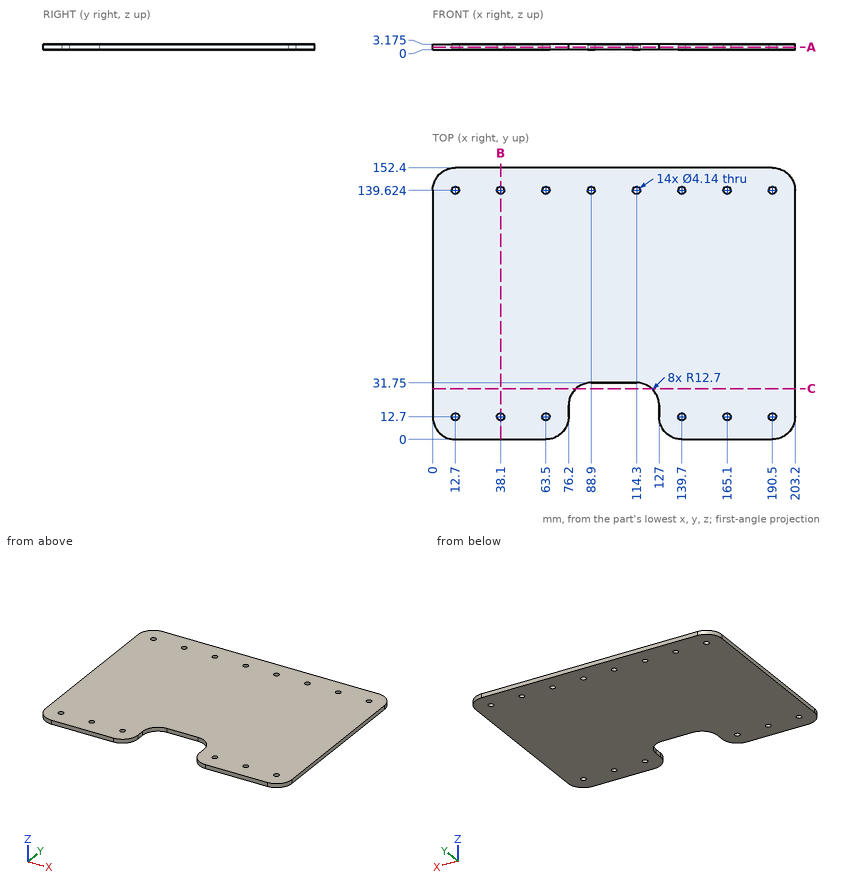
Source: three-view drawing plus pictorial views. Frame: mm from the lowest corner of the part. Round coordinates to 2 decimals unless told otherwise and drop trailing zeros. Write each loop counter-clockwise with the first axis right and the second up, starting at its lowest first coordinate (ties: lowest second). Pieces come first, ordered by that corner, then holes. Notation, with made-up numbers: M -20,34.25 L -2,34.25 A19 ccw -2,64.25 Z; hole C -29,46.25 d9. An arc over 180 degrees is marked long. One line per item, written item: value. Start each with the question number.
Item 1: Section query A-A (z = 1.35). State how many separate pieces and enclosed holes the cut face has, plus the area to 3 significant figures.
Item 2: Section query C-C (y = 28.5). Return the cut outline in (x, z) (1 decimal).
Item 3: Section query B-B (x = 38.1). Return the cut outline in (y, z) (1 decimal).
Item 4: Ray query, L1, parallel to Y at x = 190.5, z = 1.15; L2, parallel to Y at x = 88.9, z = 1.5; L3, parallel to Y at x = 39, z = 0.1 (1 decimal). Return the intervals inside material, ascending. Write a range as from..to.
Result set:
1. separate pieces: 1
1. enclosed holes: 14
1. area: 29,000 mm²
2. outline: M 0,0 L 80.4,0 L 80.4,3.2 L 0,3.2 Z; M 122.8,0 L 203.2,0 L 203.2,3.2 L 122.8,3.2 Z
3. outline: M 0,0 L 10.6,0 L 10.6,3.2 L 0,3.2 Z; M 14.8,0 L 137.6,0 L 137.6,3.2 L 14.8,3.2 Z; M 141.7,0 L 152.4,0 L 152.4,3.2 L 141.7,3.2 Z
4. L1: y = 0..10.63, 14.77..137.55, 141.69..152.4
4. L2: y = 31.75..137.55, 141.69..152.4
4. L3: y = 0..10.8, 14.6..137.8, 141.5..152.4
